Part model, mm, in its own coordinate system. Face numbers are marked on the shaded views. A direction names the side the tool comes from. Give positions to 0.01 mm unless a question says otherwise; leave off trailing zeros. Order: outer loops, then holes, each group sorted by start corner. A loop starts at its lowest first (then second) coordinate and runs counter-clockwise, first axis right, second up.
1. Slice it at D-D on x = 12. List the corners of the cut face in (y, z), and give its area (3 significant figures).
2. Slice it at A-A on y = 3.65. List the corners of the cut face in (x, z), and give its area (3 significant figures).
3. Slice it at C-C on y = 0.8. List the corners of the cut face in (x, z), and give its area (3 significant figures).
4. Which spindle directions (+Z, -Z, +X, -X, +Y, -Y) get a long thin tool onto all of the face, cutting with end or side? Do the marked faces 1 and 2. Say none if no direction does.
5. Slice it at B-B on z = -6.5. List the corners of the cut face in (x, y), and give its area (3 significant figures).
6. Drop flat-ended pins along their axis: pin 1 Ø1.3 at (x, z) = (20, -20) entering from -Y; pin 2 Ø1 at (y, z) = (1.5, -6) entering from +X; pin 3 Ø1.5 at (x, y) = (20, 2.5) entering from +Z. Give the stop position or say it passes through.
7. Probe line 1 (Z direction, x = 20, y = 2.6); line 2 (Z direction, x = 18, y = 4); line 3 (Y direction, x = 12.5, z = -21.5). List the from-to ranges inside material, lowest first.
8. Mould opens along X. For the marked faces 3, 4, 5 and 6 say: +X half, -X half, draft (parallel to the pull), parting line (faces both ways), or undercut.
from build123d import *

# Parameters (mm, degrees)
BOSS_EXTRUDE1_DEPTH  = 3.2
SKETCH2_R            = 2.4
BOSS_EXTRUDE2_DEPTH  = 1.6
LPATTERN1_COUNT      = 2
LPATTERN1_PITCH      = 8
LPATTERN1_COUNT_DIR2 = 2
LPATTERN1_PITCH_DIR2 = 8
SHELL1_T             = -1.6


with BuildPart() as part:
    # Sketch1 → Boss-Extrude1 (new body)
    with BuildSketch(Plane(origin=(0, 0, 0), x_dir=(1, 0, 0), z_dir=(0, 1, 0))):
        Polygon((0, 0), (8, 24), (24, 24), (32, 0), (24, 0), (24, 8), (8, 8), (8, 0), align=None)
    extrude(amount=BOSS_EXTRUDE1_DEPTH)

    # Sketch2 → Boss-Extrude2 (add)
    with BuildSketch(Plane(origin=(0, 3.2, 0), x_dir=(1, 0, 0), z_dir=(0, 1, 0))):
        with Locations(Location((12, 20, 0), (0, 0, 270))):
            Circle(SKETCH2_R)
    boss_extrude2 = extrude(amount=BOSS_EXTRUDE2_DEPTH)

    # LPattern1: Boss-Extrude2 2 × 2
    with Locations(*[(i * LPATTERN1_PITCH, 0, j * LPATTERN1_PITCH_DIR2) for i in range(LPATTERN1_COUNT) for j in range(LPATTERN1_COUNT_DIR2) if (i, j) != (0, 0)]):
        add(boss_extrude2)

    # Shell1
    shell1_openings = [part.faces().sort_by_distance(p)[0] for p in [
        (16, 0, -12.571428571),
    ]]
    offset(amount=SHELL1_T, openings=shell1_openings, kind=Kind.INTERSECTION)


solid = part.part
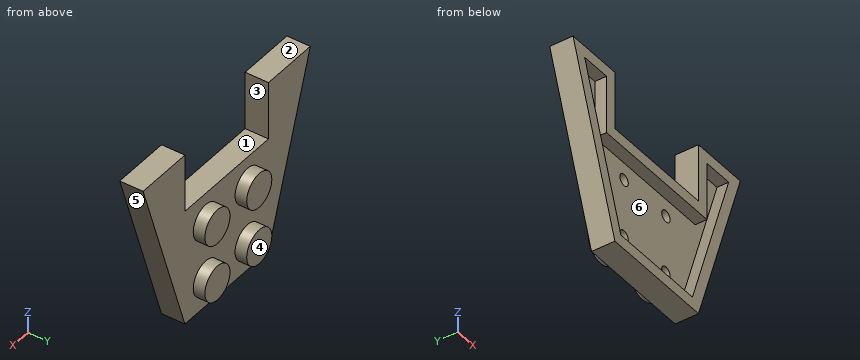
Data:
1. outline: (0, -24) - (3.2, -24) - (3.2, -22.4) - (4.8, -22.4) - (4.8, -17.6) - (3.2, -17.6) - (3.2, -14.4) - (4.8, -14.4) - (4.8, -9.6) - (3.2, -9.6) - (3.2, -8) - (0, -8) - (0, -9.6) - (1.6, -9.6) - (1.6, -11.2) - (3.2, -11.2) - (3.2, -12.8) - (1.6, -12.8) - (1.6, -19.2) - (3.2, -19.2) - (3.2, -20.8) - (1.6, -20.8) - (1.6, -22.4) - (0, -22.4) - close
1. area: 41.0 mm2
2. outline: circle Ø4.8 at (12, -20); circle Ø4.8 at (12, -12); circle Ø4.8 at (20, -20); circle Ø4.8 at (20, -12)
2. area: 72.4 mm2
3. outline: (0, 0) - (8, -24) - (24, -24) - (32, 0) - (24, 0) - (24, -8) - (8, -8) - (8, 0) - close; hole (2.22, -1.6) - (9.15, -22.4) - (22.85, -22.4) - (29.78, -1.6) - (25.6, -1.6) - (25.6, -9.6) - (6.4, -9.6) - (6.4, -1.6) - close
3. area: 173 mm2
4. face 1: +Z, +Y, -Y
4. face 2: +Z, +X, -X, +Y, -Y
5. outline: (2.17, 0) - (3.85, 0) - (3.85, 1.6) - (6.4, 1.6) - (6.4, 0) - (8, 0) - (8, 3.2) - (2.17, 3.2) - close; (24, 0) - (25.6, 0) - (25.6, 1.6) - (28.15, 1.6) - (28.15, 0) - (29.83, 0) - (29.83, 3.2) - (24, 3.2) - close
5. area: 29.2 mm2
6. pin 1: stops at y = 3.2
6. pin 2: stops at x = 30.17
6. pin 3: stops at z = -8
7. line 1: z = -24 to -20.8, -19.2 to -12.8, -11.2 to -8
7. line 2: z = -21.33 to -18.67, -13.33 to -10.67
7. line 3: y = 1.6 to 4.8
8. face 3: undercut
8. face 4: draft
8. face 5: +X half
8. face 6: undercut
